Autodesk Inventor part; units mm, degrees
ref_plane "YZ Plane" through (0, 0, 0) normal (1, 0, 0) x (0, 1, 0)
ref_plane "XZ Plane" through (0, 0, 0) normal (0, 1, 0) x (-1, 0, 0)
ref_plane "XY Plane" through (0, 0, 0) normal (0, 0, 1) x (1, 0, 0)
sketch "Sketch1" plane through (0, 0, 0) normal (0, 0, 1) x (1, 0, 0)
  line L0 (0, 0) -> (25.4, 0)
  line L1 (25.4, 0) -> (25.4, 50.8)
  line L2 (25.4, 50.8) -> (0, 50.8)
  line L3 (0, 50.8) -> (0, 0)
  line L4 (3.175, 3.175) -> (22.225, 3.175)
  line L5 (22.225, 3.175) -> (22.225, 47.625)
  line L6 (22.225, 47.625) -> (3.175, 47.625)
  line L7 (3.175, 47.625) -> (3.175, 3.175)
  dimension "d0" = 50.8
  dimension "d1" = 25.4
  dimension "d2" = 3.175
  dimension "d3" = 3.175
  dimension "d4" = 3.175
  dimension "d5" = 3.175
extrude "Extrusion1" add sketch "Sketch1" along normal blind 127
sketch "Sketch4" plane through (25.4, 0, 0) normal (1, 0, 0) x (0, 0, -1)
  line L0 (0, 0) -> (-127, 0)
  line L1 (0, 0) -> (0, 50.8)
  line L2 (0, 50.8) -> (-127, 50.8)
  line L3 (0, 50.8) -> (0, 0)
  line L4 (-127, 50.8) -> (0, 50.8)
  line L5 (-127, 0) -> (-127, 50.8)
  line L6 (-127, 0) -> (0, 0)
  line L7 (-55.7727, 44.45) -> (-74.93, 12.5211)
  line L8 (-74.93, 6.35) -> (-52.07, 44.45) construction
  line L9 (-120.65, 6.35) -> (-6.35, 6.35)
  line L10 (-6.35, 44.45) -> (-120.65, 44.45)
  line L11 (-52.07, 38.2789) -> (-71.2273, 6.35)
  line L12 (-52.07, 44.45) -> (-29.21, 6.35) construction
  line L13 (-48.3673, 44.45) -> (-29.21, 12.5211)
  line L14 (-94.0873, 44.45) -> (-74.93, 12.5211)
  line L15 (-97.79, 44.45) -> (-74.93, 6.35) construction
  line L16 (-78.6327, 6.35) -> (-97.79, 38.2789)
  line L17 (-52.07, 38.2789) -> (-32.9127, 6.35)
  line L18 (-116.9473, 6.35) -> (-97.79, 38.2789)
  line L19 (-120.65, 44.45) -> (-120.65, 6.35)
  line L20 (-120.65, 6.35) -> (-97.79, 44.45) construction
  line L21 (-120.65, 12.5211) -> (-101.4927, 44.45)
  line L22 (-29.21, 12.5211) -> (-10.0527, 44.45)
  line L23 (-25.5073, 6.35) -> (-6.35, 38.2789)
  line L24 (-6.35, 6.35) -> (-6.35, 44.45)
  line L25 (-29.21, 6.35) -> (-6.35, 44.45) construction
  line L26 (-127, 50.8) -> (-127, 0)
  dimension "d20" = 30.964
  dimension "d21" = 61.928
  dimension "d22" = 61.928
  dimension "d23" = 61.928
  dimension "d24" = 61.928
  dimension "d25" = 3.175
  dimension "d26" = 3.175
  dimension "d27" = 3.175
  dimension "d28" = 3.175
  dimension "d29" = 3.175
  dimension "d30" = 3.175
  dimension "d31" = 3.175
  dimension "d32" = 3.175
  dimension "d33" = 3.175
  dimension "d34" = 3.175
  dimension "d35" = 6.35
  dimension "d36" = 6.35
  dimension "d37" = 6.35
  dimension "d38" = 6.35
extrude "Extrusion5" cut sketch "Sketch4" against normal blind 3.175 contours L7 L14 L10 | L10 L22 L13 | L21 L19 L10 | L24 L9 L23 | L18 L16 L9 | L9 L11 L17
sketch "Sketch5" plane through (0, 0, 0) normal (-1, 0, 0) x (0, 0, 1)
  line L0 (127, 0) -> (127, 50.8)
  line L1 (0, 50.8) -> (127, 50.8)
  line L2 (0, 50.8) -> (0, 0)
  line L3 (0, 0) -> (127, 0)
  line L4 (0, 0) -> (0, 50.8)
  line L5 (127, 0) -> (0, 0)
  line L6 (127, 50.8) -> (127, 0)
  line L7 (127, 50.8) -> (0, 50.8)
  line L8 (74.93, 38.2789) -> (55.7727, 6.35)
  line L9 (71.2273, 44.45) -> (52.07, 12.5211)
  line L10 (52.07, 6.35) -> (74.93, 44.45) construction
  line L11 (6.35, 6.35) -> (120.65, 6.35)
  line L12 (120.65, 44.45) -> (6.35, 44.45)
  line L13 (74.93, 44.45) -> (97.79, 6.35) construction
  line L14 (74.93, 38.2789) -> (94.0873, 6.35)
  line L15 (97.79, 12.5211) -> (116.9473, 44.45)
  line L16 (97.79, 6.35) -> (120.65, 44.45) construction
  line L17 (120.65, 6.35) -> (120.65, 44.45)
  line L18 (101.4927, 6.35) -> (120.65, 38.2789)
  line L19 (78.6327, 44.45) -> (97.79, 12.5211)
  line L20 (32.9127, 44.45) -> (52.07, 12.5211)
  line L21 (29.21, 44.45) -> (52.07, 6.35) construction
  line L22 (10.0527, 6.35) -> (29.21, 38.2789)
  line L23 (6.35, 44.45) -> (6.35, 6.35)
  line L24 (6.35, 6.35) -> (29.21, 44.45) construction
  line L25 (6.35, 12.5211) -> (25.5073, 44.45)
  line L26 (48.3673, 6.35) -> (29.21, 38.2789)
  dimension "d41" = 30.964
  dimension "d42" = 61.928
  dimension "d43" = 61.928
  dimension "d44" = 61.928
  dimension "d45" = 61.928
  dimension "d46" = 3.175
  dimension "d47" = 3.175
  dimension "d48" = 3.175
  dimension "d49" = 3.175
  dimension "d50" = 3.175
  dimension "d51" = 3.175
  dimension "d52" = 3.175
  dimension "d53" = 3.175
  dimension "d54" = 3.175
  dimension "d55" = 3.175
  dimension "d56" = 6.35
  dimension "d57" = 6.35
  dimension "d58" = 6.35
  dimension "d59" = 6.35
extrude "Extrusion6" cut sketch "Sketch5" against normal blind 3.175 contours L14 L11 L8 | L11 L22 L26 | L18 L17 L11 | L23 L12 L25 | L15 L19 L12 | L12 L9 L20
fillet "Fillet1" radius 3.175 36 edges at (1.5875, 12.5211, 6.35) (1.5875, 44.45, 6.35) (1.5875, 44.45, 25.5073) (1.5875, 38.2789, 29.21) (1.5875, 6.35, 10.0527) (1.5875, 6.35, 48.3673) (1.5875, 44.45, 32.9127) (1.5875, 12.5211, 52.07) (1.5875, 44.45, 71.2273) (1.5875, 38.2789, 74.93) (1.5875, 6.35, 55.7727) (1.5875, 6.35, 94.0873) (1.5875, 44.45, 78.6327) (1.5875, 44.45, 116.9473) (1.5875, 12.5211, 97.79) (1.5875, 38.2789, 120.65) (1.5875, 6.35, 101.4927) (1.5875, 6.35, 120.65) (23.8125, 44.45, 120.65) (23.8125, 44.45, 101.4927) (23.8125, 12.5211, 120.65) (23.8125, 6.35, 116.9473) (23.8125, 38.2789, 97.79) (23.8125, 6.35, 78.6327) (23.8125, 12.5211, 74.93) (23.8125, 44.45, 94.0873) (23.8125, 44.45, 55.7727) (23.8125, 38.2789, 52.07) (23.8125, 6.35, 71.2273) (23.8125, 6.35, 32.9127) (23.8125, 12.5211, 29.21) (23.8125, 44.45, 48.3673) (23.8125, 44.45, 10.0527) (23.8125, 38.2789, 6.35) (23.8125, 6.35, 25.5073) (23.8125, 6.35, 6.35)
equation "\"d3\" = d2"
equation "\"d4\" = d3"
equation "\"d5\" = d4"
equation "\"d21\" = 2 * d20"
equation "\"d22\" = d21"
equation "\"d23\" = d22"
equation "\"d24\" = d23"
equation "\"d26\" = d25"
equation "\"d27\" = d26"
equation "\"d28\" = d27"
equation "\"d29\" = d28"
equation "\"d30\" = d29"
equation "\"d31\" = d30"
equation "\"d32\" = d30"
equation "\"d33\" = d32"
equation "\"d34\" = d33"
equation "\"d42\" = 2 * d41"
equation "\"d43\" = d42"
equation "\"d44\" = d43"
equation "\"d45\" = d44"
equation "\"d47\" = d46"
equation "\"d48\" = d47"
equation "\"d49\" = d48"
equation "\"d50\" = d49"
equation "\"d51\" = d50"
equation "\"d52\" = d51"
equation "\"d53\" = d51"
equation "\"d54\" = d53"
equation "\"d55\" = d54"
properties part number "left fram piece 3"
Design review of the part built by this model. Coordinates are the model's own, in mm. A direction names the side the tool comes from. Coordinates: 2 decimals unless noted, no trailing zeros. Order: outer loops, then holes, each group sorted by start corner. A loop starts at its lowest first (then second) coordinate and runs counter-clockwise, first axis right, second up. Notation, with made-up numbers: M 57.25,87 L 93.25,87 A14 cw 93.25,112 Z; hole C 84,87.5 d6. An arc over 180 degrees is marked long. Answer as a JSON object with one key per item and string values. Group by question number.
1) Tool access review of faces 1 (the flat face through (24, 33, 120.65)), 2 (the cylindrical face through (23.79, 42.798, 91.265)), 3 (the flat face through (2, 44.45, 98)): name each direction out of +Z, -Z, +X, -X, +Y, -Y from which nothing blocks a thin tool from reaching the whole face with its end or side.
2) Mouldability with a two-part tool opening along Y and no side actions: class faces 4 (the flat face through (25.4, 25, 63)), 5 (the flat face through (24, 6.35, 98)) as pulls with the +Y half, pulls with the -Y half, needs draft (parallel to the pull), parting line crosses it, or undercut.
3) Add section B-B, the plane y = 46.5. Write out the cut boundary in (x, z) (3 decimals).
4) Add section C-C, the plane z = 37. Write out the cut boundary in (x, y) (3 decimals), then the cut area to 3 significant figures.
5) Add section A-A, the plane x = 20.75. Write out the cut boundary in (y, z) (3 decimals).
6) Wall thickness on L1, parallel to Y at x = 8, z = 82 (3 decimals); L2, parallel to Z at x = 3, y = 42.5; L3, parallel to X at y = 29, z = 17 (3 decimals): over which ranges is each line inside the solid? List them lowest first.
7) For pin 1 (1.6 mm diameter, centred on x = 2, y = 18, fed in from -Z), flat-tipped, find the tip position at first contact; note if it passes through.
Computed values:
{
 "1": {"face 1": "+X", "face 2": "+X, -X", "face 3": "-X"},
 "2": {"face 4": "needs draft", "face 5": "undercut"},
 "3": {"outline": "M 0,0 L 3.175,0 L 3.175,127 L 0,127 Z; M 22.225,0 L 25.4,0 L 25.4,127 L 22.225,127 Z"},
 "4": {"outline": "M 0,0 L 25.4,0 L 25.4,6.738 L 22.225,6.738 L 22.225,3.175 L 3.175,3.175 L 3.175,6.35 L 0,6.35 Z; M 0,25.296 L 3.175,25.296 L 3.175,37.638 L 0,37.638 Z; M 0,44.062 L 3.175,44.062 L 3.175,47.625 L 22.225,47.625 L 22.225,44.45 L 25.4,44.45 L 25.4,50.8 L 0,50.8 Z; M 22.225,13.162 L 25.4,13.162 L 25.4,25.504 L 22.225,25.504 Z", "area": "282 mm^2"},
 "5": {"outline": "M 0,0 L 3.175,0 L 3.175,127 L 0,127 Z; M 47.625,0 L 50.8,0 L 50.8,127 L 47.625,127 Z"},
 "6": {"L1": "y = 0 to 3.175, 47.625 to 50.8", "L2": "z = 0 to 6.6, 22.83 to 35.59, 68.55 to 81.31, 114.27 to 127", "L3": "x = 0 to 3.175, 22.225 to 25.4"},
 "7": {"pin 1": "stops at z = 0"}
}
